Design review of the part shown in the three views and the two pictorial views. Dimensions are in mm from the part's minimum x, y and z. A direction names the side the tool comes from. Give positions to 0.01 mm unless a question says otherwise; leave off trailing zeros. Write each loop counter-clockwise with the first axis right and the second up, starting at its lowest first coordinate (ties: lowest second). Pieces come first, ordered by that corner, then holes.
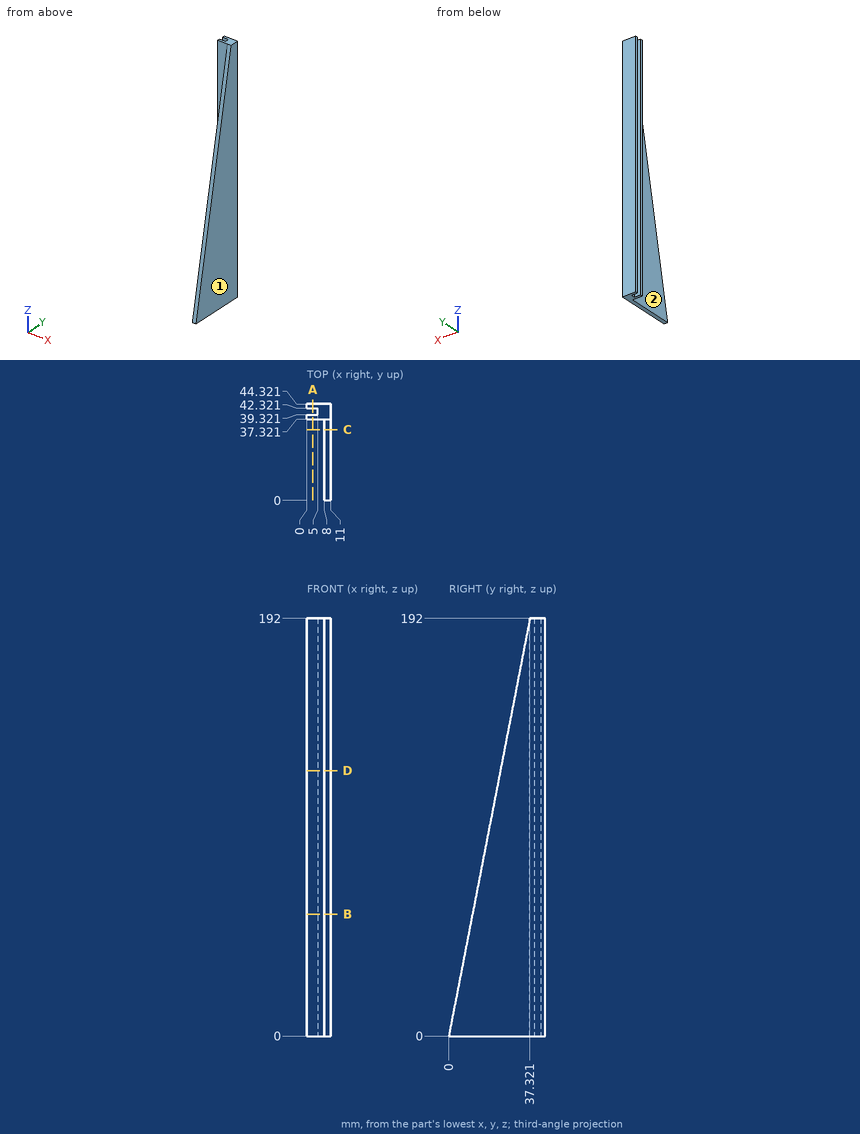
(1) To check wall thickness, follow L1, parallel to Y at x = 3.25, z = 81.5; L2, parallel to X at y = 19, z = 84; L3, parallel to Y at x = 6.75, z = 84.5. State the ranges of each line that lie inside material, in increasing order.
Resolved:
L1: y = 37.32 to 39.32, 42.32 to 44.32
L2: x = 8 to 11
L3: y = 37.32 to 44.32
(2) Consider section C-C, the plane y = 32.5. Give the boundary of the cut face in (x, z).
Resolved:
outline: (8, 0) - (11, 0) - (11, 167.2) - (8, 167.2) - close
(3) Consider section D-D, the plane z = 122. Give the boundary of the cut face in (x, y).
Resolved:
outline: (0, 37.32) - (8, 37.32) - (8, 23.71) - (11, 23.71) - (11, 44.32) - (0, 44.32) - (0, 42.32) - (5, 42.32) - (5, 39.32) - (0, 39.32) - close
(4) Clearance check with flat-ended pins moving along their axes: P1, Ø2, axis at x = 6.5, z = 83, coming from the -Y side; P2, Ø2.5, axis at y = 41, z = 61, coming from the -X side; P3, Ø18.5, axis at y = 23.5, z = 50, coming from the -X side. State where each tip first meets the part, or that it passes through.
Resolved:
P1: stops at y = 37.32
P2: stops at x = 5
P3: stops at x = 8
(5) Consider section A-A, the plane x = 2.75. Give the boundary of the cut face in (y, z), then the cut area to 3 significant figures.
Resolved:
outline: (37.32, 0) - (39.32, 0) - (39.32, 192) - (37.32, 192) - close; (42.32, 0) - (44.32, 0) - (44.32, 192) - (42.32, 192) - close
area: 768 mm2
(6) Consider section B-B, the plane z = 56. Give the boundary of the cut face in (x, y).
Resolved:
outline: (0, 37.32) - (8, 37.32) - (8, 10.89) - (11, 10.89) - (11, 44.32) - (0, 44.32) - (0, 42.32) - (5, 42.32) - (5, 39.32) - (0, 39.32) - close
(7) Tool access review of the marked faces 1 and 2: name each direction out of +Z, -Z, +X, -X, +Y, -Y from which nothing blocks a thin tool from reaching the whole face with its end or side.
Resolved:
face 1: +Z, -Z, +X, +Y, -Y
face 2: +Z, -Z, -X, -Y
